Part model, mm, in its own coordinate system. Coordinates: 2 decimals unless noted, no trailing zeros. Write each loop counter-clockwise with the first axis right and the second up, starting at its lowest first coordinate (ties: lowest second). Pieces come first, ordered by that corner, then holes. Notation, with made-up numbers: (29, 11) -> (60, 11) arc R30 ccw to (60, 49) -> close; hole circle Ø9 at (58, 52.25). An arc over 180 degrees is marked (long way). Write item = value, one per line. Start each with the question number.
Q1. Band-saw the part on A-A, the plane x = -3.5. List the corners of the cut face in (y, z).
Q2. Probe line 1 (Z direction, x = -1.25, y = 2.25); line 2 (Z direction, x = -8.75, y = 3); line 3 (Y direction, x = -0.75, z = -31). List the from-to ranges inside material, lowest first.
Q3. Pin check, flat tips, straight feed: P1, Ø6, axis at x = -7.5, z = -24, coming from the -Y side; P2, Ø1.6, axis at x = -3, z = -31, coming from the +Y side; P3, Ø3, axis at x = -1.5, z = -47, coming from the +Y side; P4, Ø1, axis at y = 1.5, z = -30.5, coming from the +X side. Stop position of each tip, or through.
Q4. Band-saw the part on B-B, the plane z = -41. List the corners of the cut face in (x, y).
Q5. Band-saw the part on C-C, the plane y = 19.5. List the corners of the cut face in (x, z).
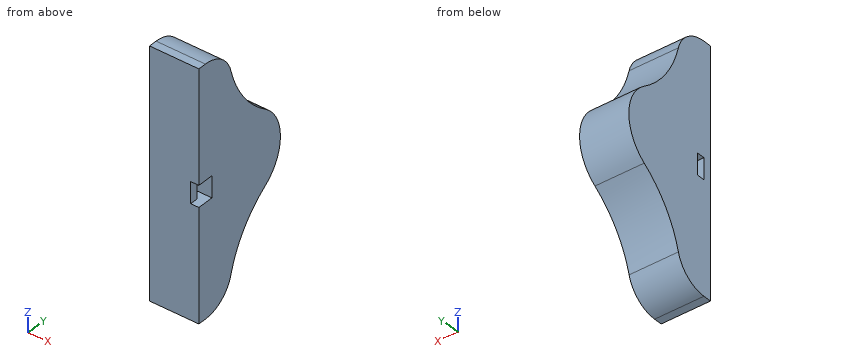
from build123d import *

# Parameters (mm, degrees)
SKETCH1_W           = 5.2
SKETCH1_H           = 2
BOSS_EXTRUDE1_DEPTH = 10
BOSS_EXTRUDE2_DEPTH = 2


with BuildPart() as part:
    # Sketch1 → Boss-Extrude1 (new body)
    with BuildSketch(Plane(origin=(0, 0, 0), x_dir=(0, 0, -1), z_dir=(1, 0, 0))):
        with BuildLine():
            Line((0, 0), (60, 0))
            Line((60, 0), (60, 2))
            ThreePointArc((60, 2), (58.327156209, 6.928038895), (54, 9.819352237))
            ThreePointArc((54, 9.819352237), (45.597676291, 13.737420129), (39.042132847, 20.292963573))
            ThreePointArc((39.042132847, 20.292963573), (30, 25), (20.957867153, 20.292963573))
            ThreePointArc((20.957867153, 20.292963573), (14.402323709, 13.737420129), (6, 9.819352237))
            ThreePointArc((6, 9.819352237), (1.672843791, 6.928038895), (0, 2))
            Line((0, 2), (0, 0))
        make_face()
        with Locations((30, 3)):
            Rectangle(SKETCH1_W, SKETCH1_H, mode=Mode.SUBTRACT)
    extrude(amount=-BOSS_EXTRUDE1_DEPTH)

    # Sketch2 → Boss-Extrude2 (add)
    with BuildSketch(Plane(origin=(0, 0, 0), x_dir=(0, 0, -1), z_dir=(1, 0, 0))):
        with BuildLine():
            Line((0, 0), (27.4, 0))
            Line((27.4, 0), (27.4, 4))
            Line((27.4, 4), (32.6, 4))
            Line((32.6, 4), (32.6, 0))
            Line((32.6, 0), (60, 0))
            Line((60, 0), (60, 2))
            ThreePointArc((60, 2), (58.327156209, 6.928038895), (54, 9.819352237))
            ThreePointArc((54, 9.819352237), (45.597676291, 13.737420129), (39.042132847, 20.292963573))
            ThreePointArc((39.042132847, 20.292963573), (30, 25), (20.957867153, 20.292963573))
            ThreePointArc((20.957867153, 20.292963573), (14.402323709, 13.737420129), (6, 9.819352237))
            ThreePointArc((6, 9.819352237), (1.672843791, 6.928038895), (0, 2))
            Line((0, 2), (0, 0))
        make_face()
    extrude(amount=BOSS_EXTRUDE2_DEPTH)


solid = part.part
Ans:
q1.outline = (0, -60) -> (2, -60) arc R8.1 ccw to (9.82, -54) arc R26.69 cw to (20.29, -39.04) arc R11.04 ccw to (20.29, -20.96) arc R26.69 cw to (9.82, -6) arc R8.1 ccw to (2, 0) -> (0, 0) -> close; hole (2, -32.6) -> (4, -32.6) -> (4, -27.4) -> (2, -27.4) -> close
q2.line_1 = -60 to -32.6, -27.4 to 0
q2.line_2 = -59.94 to -32.6, -27.4 to -0.06
q2.line_3 = 0 to 2, 4 to 24.95
q3.P1 = 0
q3.P2 = 25
q3.P3 = 13.81
q3.P4 = 0
q4.outline = (-10, 0) -> (2, 0) -> (2, 17.82) -> (-10, 17.82) -> close
q5.outline = (-10, -39.62) -> (2, -39.62) -> (2, -20.38) -> (-10, -20.38) -> close
